Autodesk Inventor part; units mm, degrees
ref_plane "YZ Plane" through (0, 0, 0) normal (1, 0, 0) x (0, 1, 0)
ref_plane "XZ Plane" through (0, 0, 0) normal (0, 1, 0) x (-1, 0, 0)
ref_plane "XY Plane" through (0, 0, 0) normal (0, 0, 1) x (1, 0, 0)
sketch "Sketch1" plane through (0, 0, 0) normal (0, 0, 1) x (1, 0, 0)
  line L0 (0, 0) -> (0, 25)
  line L1 (0, 25) -> (165, 25)
  line L2 (165, 0) -> (0, 0)
  line L3 (190, 0) -> (190, -165)
  line L4 (190, -165) -> (165, -165)
  line L5 (165, -165) -> (165, 0)
  line L6 (165, 25) -> (180, 25)
  line L7 (190, 15) -> (190, 0)
  circle A0 centre (10, 12.5) radius 1.5
  circle A1 centre (177.5, -155) radius 1.5
  circle A2 centre (179, 12.5) radius 1.5
  arc A3 (190, 23) -> (188, 25) centre (188, 23) ccw
  arc A4 (190, 15) -> (180, 25) centre (180, 15) ccw
  dimension "d0" = 25
  dimension "d1" = 165
  dimension "d2" = 25
  dimension "d3" = 165
  dimension "d6" = 3
  dimension "d7" = 3
  dimension "d8" = 3
  dimension "d9" = 2
  dimension "d10" = 10
extrude "Extrusion1" add sketch "Sketch1" along normal blind 25
properties part number "l almini"
Work out the finished part from the listing and answer in its coordinate system (mm). A direction names the side the tool comes from. Round coordinates to 2 decimals unless told otherwise and drop trailing zeros. Write each loop counter-clockwise with the first axis right and the second up, starting at its lowest first coordinate (ties: lowest second). Pieces come first, ordered by that corner, then holes. Notation, with made-up numbers: (84.5, -12) -> (106.5, -12) arc R25 cw to (106.5, 11) -> close; hole circle Ø4 at (51, 85). An arc over 180 degrees is marked (long way). Answer as CSV lines item,"result". Start each with the question number.
(1) Each of these flat-tipped pins is pushed along its axis until it touches: pin 1 (4 mm diameter, centred on x = 77, y = -3.5, fed in from -Z); pin 2 (12.5 mm diameter, centred on x = 71.5, z = 6.5, fed in from -Y). Where does it stop, or does it pass through?
(2) A tool of negligible diameter and unlimited length cuts with its end or side. For faces 1 (the flat face through (130, 8, 0)), 2 (the flat face through (84, 0, 12)), from which of +Z, -Z, +X, -X, +Y, -Y can it reach the whole face along a straight path? Write none if from no direction.
(3) The part is cut by section B-B, the plane y = -8.5. Give the vertices of the cut face in (x, z).
(4) The part is cut by section C-C, the plane x = 105. Give the vertices of the cut face in (y, z).
(5) Find the intervals of material crossed by probe 1 along Y at (x, z) = (10, 15.5); probe 2 along X at (y, z) = (-155, 9); probe 3 along X at (y, z) = (-146.5, 11), in increasing order.
(6) The part is cut by section A-A, the plane z = 12.75. Give the vertices of the cut face in (x, y).
Output values:
1,pin 1,"passes through"
1,pin 2,"stops at y = 0"
2,face 1,"-Z, +X, -X, +Y, -Y"
2,face 2,"+Z, -Z, -X, -Y"
3,outline,"(165, 0) -> (190, 0) -> (190, 25) -> (165, 25) -> close"
4,outline,"(0, 0) -> (25, 0) -> (25, 25) -> (0, 25) -> close"
5,probe 1,"y = 0 to 11, 14 to 25"
5,probe 2,"x = 165 to 176, 179 to 190"
5,probe 3,"x = 165 to 190"
6,outline,"(0, 0) -> (165, 0) -> (165, -165) -> (190, -165) -> (190, 15) arc R10 ccw to (180, 25) -> (0, 25) -> close; hole circle Ø3 at (10, 12.5); hole circle Ø3 at (177.5, -155); hole circle Ø3 at (179, 12.5)"
